Here's how the part is built. I have some questions about the finished solid (model axes, mm). A direction names the side the tool comes from. Coordinates: 2 decimals unless noted, no trailing zeros. Loops run counter-clockwise (first coordinate to the right, second up) from the corner with the lowest first, then second, coordinate; pieces in that order, holes last.
```python
from build123d import *

# Parameters (mm, degrees)
SKETCH1_R           = 8
BOSS_EXTRUDE1_DEPTH = 158
SKETCH2_R           = 19.5
BOSS_EXTRUDE2_DEPTH = 10
SKETCH3_R           = 10
SKETCH3_R_2         = 0.8
CUT_EXTRUDE1_DEPTH  = 2
SKETCH3_2_R         = 0.8
CUT_EXTRUDE2_DEPTH  = 8


with BuildPart() as part:
    # Sketch1 → Boss-Extrude1 (new body)
    with BuildSketch(Plane.XY):
        Circle(SKETCH1_R)
    extrude(amount=BOSS_EXTRUDE1_DEPTH)

    # Sketch2 → Boss-Extrude2 (add)
    with BuildSketch(Plane.XY.offset(158)):
        Circle(SKETCH2_R)
    extrude(amount=-BOSS_EXTRUDE2_DEPTH)

    # Sketch3 → Cut-Extrude1 (cut)
    with BuildSketch(Plane.XY.offset(158)):
        Circle(SKETCH3_R)
        with Locations((6.84496079, 1.465097875)):
            Circle(SKETCH3_R_2, mode=Mode.SUBTRACT)
        with Locations((-1.465097875, 6.84496079)):
            Circle(SKETCH3_R_2, mode=Mode.SUBTRACT)
        with Locations((-6.84496079, -1.465097875)):
            Circle(SKETCH3_R_2, mode=Mode.SUBTRACT)
        with Locations((1.465097875, -6.84496079)):
            Circle(SKETCH3_R_2, mode=Mode.SUBTRACT)
    extrude(amount=-CUT_EXTRUDE1_DEPTH, mode=Mode.SUBTRACT)

    # Sketch3<2> → Cut-Extrude2 (cut)
    with BuildSketch(Plane.XY.offset(158)):
        with Locations((6.84496079, 1.465097875)):
            Circle(SKETCH3_2_R)
        with Locations((-1.465097875, 6.84496079)):
            Circle(SKETCH3_2_R)
        with Locations((-6.84496079, -1.465097875)):
            Circle(SKETCH3_2_R)
        with Locations((1.465097875, -6.84496079)):
            Circle(SKETCH3_2_R)
    extrude(amount=-CUT_EXTRUDE2_DEPTH, mode=Mode.SUBTRACT)


solid = part.part
```
1. I want a section at A-A (z = 36). Please give me the cut outline in (x, y).
2. I want a section at B-B (x = 14.5). Please give me the cut outline in (y, z).
3. On a 3-axis mill with a long thin cutter (end or side, diameter ignored), from which of +Z, -Z, +X, -X, +Y, -Y can I reach the whole of each face in a straight line? I mean faces 5 (the flat face through (8.4, 0.3, 148)), 6 (the flat face through (0, 0, 0)). Say none if no direction works.
4. For pin 1 (1.8 mm diameter, centred on x = -7, y = -1, fed in from +Z); pin 2 (2 mm diameter, centred on y = 4.5, z = 77.5, fed in from -X); pin 3 (12 mm diameter, centred on y = -0.5, z = 41.5, fed in from +X), each with a flat end and sliding along its axis, tell me the tip position at first contact or that it passes through.
5. We'd pull the mould along Y, two halves only. Please class faces 1 (the flat face through (0, 0, 156)), 2 (the cylindrical face through (-2.17, -9.76, 157.01)), 3 (the flat face through (-9, 5, 158)), 4 (the cylindrical face through (-1.73, -7.81, 72.96)): +Y half, -Y half, draft (parallel to the pull), parting line (faces both ways), or undercut.
6. I need wall thicknesses on line 1 along Z through (x, y) = (-13, 9.5); line 2 along Z through (x, y) = (-3, 1); line 3 along X through (y, z) = (-1, 59). Which ranges of each line are inside material? Lowest first, please.
Response values:
1. outline: circle Ø16 at (0, 0)
2. outline: (-13.04, 148) - (13.04, 148) - (13.04, 158) - (-13.04, 158) - close
3. face 5: -Z
3. face 6: -Z, +X, -X, +Y, -Y
4. pin 1: stops at z = 156
4. pin 2: stops at x = -7.19
4. pin 3: stops at x = 8
5. face 1: undercut
5. face 2: undercut
5. face 3: draft
5. face 4: parting line
6. line 1: z = 148 to 158
6. line 2: z = 0 to 156
6. line 3: x = -7.94 to 7.94
